Here's how the part is built. I have some questions about the finished solid (model axes, mm). Face numbers are marked on the shaded views. A direction names the side the tool comes from. Round coordinates to 2 decimals unless told otherwise and drop trailing zeros. Loops run counter-clockwise (first coordinate to the right, second up) from the corner with the lowest first, then second, coordinate; pieces in that order, holes last. Notation, with made-up numbers: M -6,71 L 2,71 A19 cw 2,78 Z; hole C -26,-25.5 d2. An arc over 180 degrees is marked long. Use a Markdown table: item, result.
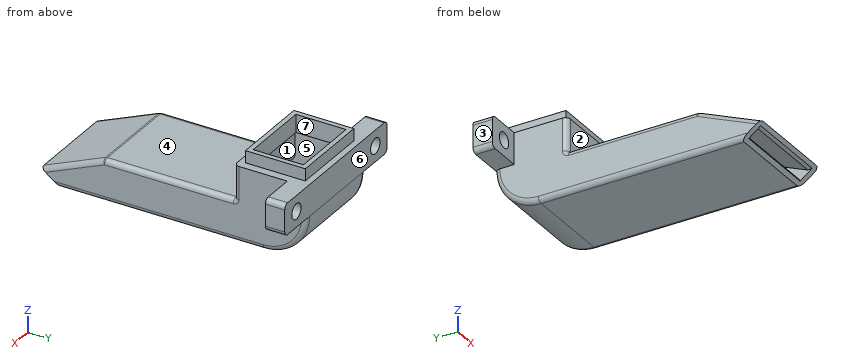
```python
from build123d import *

# Parameters (mm, degrees)
CYLINDER037_R          = 1.6
CYLINDER037_DEPTH      = 30
CYLINDER037_ROLL_ANGLE = -90
CYLINDER036_R          = 1.6
CYLINDER036_DEPTH      = 30
CYLINDER036_ROLL_ANGLE = -90
BOX034_W               = 8.25
BOX034_H               = 4
BOX034_DEPTH           = 6.5
BOX035_W               = 8.25
BOX035_H               = 4
BOX035_DEPTH           = 6.5
FILLET028_R            = 1
BOX037_W               = 14.6
BOX037_H               = 10.4
BOX037_DEPTH           = 12
BOX036_W               = 16.6
BOX036_H               = 12.4
BOX036_DEPTH           = 3
PAD012_DEPTH           = 20
FILLET029_1_R          = 9
FILLET029_2_R          = 0.2
THICKNESS001_T         = -1.2
CHAMFER009_1_SIZE      = 1
CHAMFER009_2_SIZE      = 0.5
FILLET030_R            = 1
CHAMFER010_SIZE        = 0.3


with BuildPart() as cylinder037:
    # Cylinder037 → Cylinder037 (new body)
    with BuildSketch(Plane.XY):
        Circle(CYLINDER037_R)
    extrude(amount=CYLINDER037_DEPTH)


with BuildPart() as cylinder037_1:
    # Cylinder037 roll: moved
    add(cylinder037.part.rotate(Axis((0, 0, 0), (1, 0, 0)), CYLINDER037_ROLL_ANGLE))


with BuildPart() as cylinder037_2:
    # Cylinder037 placement: moved
    add(cylinder037_1.part.moved(Location((-25, 27, -34.75))))


with BuildPart() as fusion033:
    # Cylinder036 → Cylinder036 (new body)
    with BuildSketch(Plane.XY):
        Circle(CYLINDER036_R)
    extrude(amount=CYLINDER036_DEPTH)


with BuildPart() as fusion033_1:
    # Cylinder036 roll: moved
    add(fusion033.part.rotate(Axis((0, 0, 0), (1, 0, 0)), CYLINDER036_ROLL_ANGLE))


with BuildPart() as fusion033_2:
    # Cylinder036 placement: moved
    add(fusion033_1.part.moved(Location((2, 27, -34.75))))

    # Fusion033: union Cylinder037
    add(cylinder037_2.part)


with BuildPart() as cube034:
    # Box034 → Box034 (new body)
    with BuildSketch(Plane(origin=(-29, 45, -38), x_dir=(1, 0, 0), z_dir=(0, 0, 1))):
        with Locations((4.125, 2)):
            Rectangle(BOX034_W, BOX034_H)
    extrude(amount=BOX034_DEPTH)


with BuildPart() as fillet028:
    # Box035 → Box035 (new body)
    with BuildSketch(Plane(origin=(-2.25, 45, -38), x_dir=(1, 0, 0), z_dir=(0, 0, 1))):
        with Locations((4.125, 2)):
            Rectangle(BOX035_W, BOX035_H)
    extrude(amount=BOX035_DEPTH)

    # Fusion032: union Cube034
    add(cube034.part)

    # Cut039: cut Fusion033
    add(fusion033_2.part, mode=Mode.SUBTRACT)

    # Fillet028
    fillet028_edges = [fillet028.edges().sort_by_distance(p)[0] for p in [
        (6, 47, -31.5),
        (6, 47, -38),
        (-29, 47, -31.5),
        (-29, 47, -38),
    ]]
    fillet(fillet028_edges, radius=FILLET028_R)


with BuildPart() as cube037:
    # Box037 → Box037 (new body)
    with BuildSketch(Plane(origin=(-18.8, 36.3, -39), x_dir=(1, 0, 0), z_dir=(0, 0, 1))):
        with Locations((7.3, 5.2)):
            Rectangle(BOX037_W, BOX037_H)
    extrude(amount=BOX037_DEPTH)


with BuildPart() as cube036:
    # Box036 → Box036 (new body)
    with BuildSketch(Plane(origin=(-19.8, 35.3, -32), x_dir=(1, 0, 0), z_dir=(0, 0, 1))):
        with Locations((8.3, 6.2)):
            Rectangle(BOX036_W, BOX036_H)
    extrude(amount=BOX036_DEPTH)


with BuildPart() as chamfer010:
    # Sketch014 → Pad012 (new body)
    with BuildSketch(Plane(origin=(-1.5, 4, 0), x_dir=(0, 1, 0), z_dir=(1, 0, 0))):
        Polygon((-10, -44), (2.97206, -38.5), (30, -38.5), (30, -31.5), (45, -31.5), (45, -47), (-6, -47), align=None)
    extrude(amount=-PAD012_DEPTH)

    # Fillet029 1
    fillet029_1_edges = [chamfer010.edges().sort_by_distance(p)[0] for p in [
        (-11.5, 49, -47),
    ]]
    fillet(fillet029_1_edges, radius=FILLET029_1_R)

    # Fillet029 2
    fillet029_2_edges = [chamfer010.edges().sort_by_distance(p)[0] for p in [
        (-11.5, 34, -38.5),
    ]]
    fillet(fillet029_2_edges, radius=FILLET029_2_R)

    # Thickness001
    thickness001_openings = [chamfer010.faces().sort_by_distance(p)[0] for p in [
        (-11.5, -4, -45.5),
    ]]
    offset(amount=THICKNESS001_T, openings=thickness001_openings)

    # Fusion034: union Cube036
    add(cube036.part)

    # Cut040: cut Cube037
    add(cube037.part, mode=Mode.SUBTRACT)

    # Chamfer009 1
    chamfer009_1_edges = [chamfer010.edges().sort_by_distance(p)[0] for p in [
        (-11.5, -3.6, -45.8),
    ]]
    chamfer(chamfer009_1_edges, length=CHAMFER009_1_SIZE)

    # Chamfer009 2
    chamfer009_2_edges = [chamfer010.edges().sort_by_distance(p)[0] for p in [
        (-11.5, -4.889764, -44.832677),
    ]]
    chamfer(chamfer009_2_edges, length=CHAMFER009_2_SIZE)

    # Fusion035: union Fillet028
    add(fillet028.part)

    # Fillet030
    fillet030_edges = [chamfer010.edges().sort_by_distance(p)[0] for p in [
        (-1.5, 19, -47),
        (-21.5, 19, -47),
        (-1.5, 0.48603, -41.25),
        (-1.5, 20.38603, -38.5),
        (-11.5, 6.97206, -38.5),
        (-21.5, 0.48603, -41.25),
        (-21.5, 20.38603, -38.5),
    ]]
    fillet(fillet030_edges, radius=FILLET030_R)

    # Chamfer010
    chamfer010_edges = [chamfer010.edges().sort_by_distance(p)[0] for p in [
        (-11.5, -2.6, -45.8),
    ]]
    chamfer(chamfer010_edges, length=CHAMFER010_SIZE)


solid = chamfer010.part
```
Q1. Will these pins go through, and if not, where does the flat tip stop? P1, Ø5.5, axis at x = -8.5, z = -35.5, coming from the -Y side; P2, Ø3, axis at x = -8, y = 20, coming from the +Z side; P3, Ø0.8, axis at y = 41, z = -30.5, coming from the -X side; P4, Ø3, axis at x = -25, z = -34.75, coming from the -Y side.
Return value:
| item | result |
|---|---|
| P1 | stops at y = 34 |
| P2 | stops at z = -38.5 |
| P3 | stops at x = -19.8 |
| P4 | passes through |
Q2. Imagine slicing it at C-C, the plane y = 18.5. Please give me the cut outline in (x, z).
Return value:
| item | result |
|---|---|
| outline | M -21.5,-46 A1 ccw -20.5,-47 L -2.5,-47 A1 ccw -1.5,-46 L -1.5,-39.5 A1 ccw -2.5,-38.5 L -20.5,-38.5 A1 ccw -21.5,-39.5 Z; hole M -20.3,-45.8 L -2.7,-45.8 L -2.7,-39.7 L -20.3,-39.7 Z |
Q3. For the marked faces 4, 5, 6 and 7, which set-ups out of +Z, -Z, +X, -X, +Y, -Y let a thin tool reach every point of the face, with its end or its side?
Return value:
| item | result |
|---|---|
| face 4 | +Z, +X, -X, -Y |
| face 5 | none |
| face 6 | +Z, -Z, +X, -X, +Y |
| face 7 | +Z |
Q4. Imagine slicing it at A-A, the plane z = -34.75. Please give me the cut outline in (x, y).
Return value:
| item | result |
|---|---|
| outline | M -29,45 L -26.6,45 L -26.6,49 L -29,49 Z; M -23.4,45 L -21.5,45 L -21.5,35 A1 ccw -20.5,34 L -2.5,34 A1 ccw -1.5,35 L -1.5,45 L 0.4,45 L 0.4,49 L -23.4,49 Z; M 3.6,45 L 6,45 L 6,49 L 3.6,49 Z; hole M -20.3,35.2 L -2.7,35.2 L -2.7,47.8 L -20.3,47.8 Z |
Q5. Imagine slicing it at D-D, the plane z = -29.75. Please give me the cut outline in (x, y), then the cut area to 3 significant figures.
Return value:
| item | result |
|---|---|
| outline | M -19.8,35.3 L -3.2,35.3 L -3.2,47.7 L -19.8,47.7 Z; hole M -18.8,36.3 L -4.2,36.3 L -4.2,46.7 L -18.8,46.7 Z |
| area | 54.0 mm^2 |
Q6. I need wall thicknesses on line 1 (X direction, y = 35.5, z = -34.75); line 2 (Z direction, x = -4, y = 26.5); line 3 (Z direction, x = 2, y = 47). Which ranges of each line are inside material? Lowest first, please. Write a range as from..to.
Return value:
| item | result |
|---|---|
| line 1 | x = -21.5..-20.3, -2.7..-1.5 |
| line 2 | z = -47..-45.8, -39.7..-38.5 |
| line 3 | z = -38..-36.35, -33.15..-31.5 |
Q7. We'd pull the mould along X, two halves only. Please class the marked faces 1, 2 and 3: pulls with the +X half, pulls with the -X half, needs draft (parallel to the pull), parting line crosses it, or undercut.
Return value:
| item | result |
|---|---|
| face 1 | undercut |
| face 2 | needs draft |
| face 3 | pulls with the -X half |
